```python
from build123d import *

# Parameters (mm, degrees)
FILLET_1_R          = 0.3
FILLET_2_R          = 0.8
FILLET_3_R          = 0.2
EXTRUDE_1_DEPTH     = 1
CUT_EXTRUDE_1_DEPTH = 2.25
CUT_EXTRUDE_2_DEPTH = 0.15
FILLET_5_R          = 0.15
FILLET_4_R          = 0.3


with BuildPart() as part:
    # 草图1 → 旋转1 (revolve)
    with BuildSketch(Plane.XY, mode=Mode.PRIVATE) as revolve_1_sk:
        Polygon((0, 2.65), (3.4, 2.65), (3.4, 0.551967957), (2.6, 0.551967957), (2.505416246, 0.412581372), (2.370117547, 0.412581372), (2.19193733, 0.15), (0, 0.15), align=None)
    revolve(revolve_1_sk.sketch.rotate(Axis((0, 2.65, 0), (0, -1, 0)), 180), axis=Axis((0, 2.65, 0), (0, -1, 0)))

    # 圆角1
    fillet_1_edges = [part.edges().sort_by_distance(p)[0] for p in [
        (3.4, 2.65, 0),
    ]]
    fillet(fillet_1_edges, radius=FILLET_1_R)

    # 圆角2
    fillet_2_edges = [part.edges().sort_by_distance(p)[0] for p in [
        (3.4, 0.551967957, 0),
    ]]
    fillet(fillet_2_edges, radius=FILLET_2_R - 0.0001)  # a hair under: the kernel refuses the full size

    # 圆角3
    fillet_3_edges = [part.edges().sort_by_distance(p)[0] for p in [
        (2.19193733, 0.15, 0),
    ]]
    fillet(fillet_3_edges, radius=FILLET_3_R)

    # 草图3 → 凸台-拉伸1 (add, symmetric)
    with BuildSketch(Plane.XY):
        Polygon((-1.798436821, 0.15), (3.65, 0.15), (3.65, 2.65), (-1.4, 2.65), (-1.4, 2.8), (3.8, 2.8), (3.8, 0.15), (5.9, 0.15), (5.9, 0), (-1.798436821, 0), align=None)
    extrude(amount=EXTRUDE_1_DEPTH, both=True)

    # 草图4 → 切除-拉伸1 (cut)
    with BuildSketch(Plane(origin=(5.9, 0, 0), x_dir=(0, 0, -1), z_dir=(1, 0, 0))):
        Polygon((-1, 1.351967957), (0.5, 0.15), (0.5, 0), (-0.5, 0), (-0.5, 0.15), (-1, 0.15), align=None)
    extrude(amount=-CUT_EXTRUDE_1_DEPTH, mode=Mode.SUBTRACT)

    # 草图5 → 切除-拉伸2 (cut)
    with BuildSketch(Plane.XZ):
        Polygon((3.65, 0.5), (2.484512448, -1), (3.65, -1), align=None)
    extrude(amount=-CUT_EXTRUDE_2_DEPTH, mode=Mode.SUBTRACT)

    # 圆角5
    fillet_5_edges = [part.edges().sort_by_distance(p)[0] for p in [
        (3.65, 2.65, 0),
        (3.8, 0.15, -0.75),
    ]]
    fillet(fillet_5_edges, radius=FILLET_5_R)

    # 圆角4
    fillet_4_edges = [part.edges().sort_by_distance(p)[0] for p in [
        (3.65, 0, -0.75),
        (3.8, 2.8, 0),
    ]]
    fillet(fillet_4_edges, radius=FILLET_4_R)


solid = part.part
```
The listing builds one solid part. Answer for the finished solid, in the listing's coordinates (mm). Round coordinates to 2 decimals unless told otherwise and drop trailing zeros. Order: outer loops, then holes, each group sorted by start corner. A loop starts at its lowest first (then second) coordinate and runs counter-clockwise, first axis right, second up. Notation, with made-up numbers: (-33, 5.5) -> (10, 5.5) arc R18 cw to (10, 20.5) -> close; hole circle Ø6 at (34, 5). An arc over 180 degrees is marked (long way). Answer as CSV lines item,"result".
Q1. Given pin 1 (4 mm diameter, centred on x = 0, z = -0.5, fed in from -Y); pin 2 (1.5 mm diameter, centred on y = 1.5, z = -2, fed in from +X), each flat-ended and moving along its own axis, determine where each tip first touches the part or whether it passes through.
Computed values:
pin 1,"stops at y = 0"
pin 2,"stops at x = 3.16"
Q2. A cutting plane is placed at D-D on y = 1.25. Determine the outline of the cut face in (x, z).
Computed values:
outline,"circle Ø6.79 at (0, 0); (3.65, -1) -> (3.8, -1) -> (3.8, 0.87) -> (3.65, 0.87) -> close"
Q3. Consider line 1 (Y direction, x = 2, z = -1.75); line 2 (Y direction, x = 1.75, z = 1.75); line 3 (X direction, y = 2.4, z = -2). Determine where each line is inside the solid, lowest interval first. Write a range as from..to.
Computed values:
line 1,"y = 0.55..2.65"
line 2,"y = 0.41..2.65"
line 3,"x = -2.74..2.74"
Q4. A cutting plane is placed at A-A on y = 2.25. Determine the outline of the cut face in (x, z), plus the area to 3 significant figures.
Computed values:
outline,"circle Ø6.8 at (0, 0); (3.65, -1) -> (3.8, -1) -> (3.8, 1) -> (3.65, 1) -> close"
area,"36.6 mm^2"
